Source: CAD feature listing. Evaluate the final solid. Frame: model axes, mm. Face numbers are marked on the shaded views. Round coordinates to 2 decimals unless told otherwise and drop trailing zeros. Order: outer loops, then holes, each group sorted by start corner. A loop starts at its lowest first (then second) coordinate and runs counter-clockwise, first axis right, second up. Notation, with made-up numbers: (65, 37.25) - (97, 37.25) arc R21 cw to (97, 45.25) - close; hole circle Ø1 at (-19, 30.5). An arc over 180 degrees is marked (long way). Put each result on its own line as item: value. Start each with the question number.
1) Line query: probe 1 along Y at (x, z) = (0, 14); probe 2 along X at (y, z) = (11, -13); probe 3 along X at (y, z) = (-3.25, 30). Output: solid intervals per line, ascending. Write a range as [from, to].
2) Contact query for flat-ended pins moving along their axis: P1, Ø8, axis at x = -0.5, z = 25.5, coming from the +Y side; P2, Ø6, axis at x = -10, y = 9, coming from the -Z side; P3, Ø1.5, axis at x = 9.5, z = 16, coming from the -Y side; P4, Ø4, axis at x = -9, z = 26, coming from the -Y side. Output: stop coordinate, or through.
3) Section A-A on x = 0. Output: boundary loops of the cut face in (y, z) (3 decimals).
4) Mould query, pull axis Y, two halves, no side actions, for the marked faces 1 and 2. Classes: +Y half, -Y half, draft (parallel to the pull), parting line (faces both ways), or undercut.
5) Section C-C on z = 19. Output: boundary loops of the cut face in (x, y), then the cut area to 3 significant figures.
Autodesk Inventor part; units mm, degrees
ref_plane "YZ Plane" through (0, 0, 0) normal (1, 0, 0) x (0, 1, 0)
ref_plane "XZ Plane" through (0, 0, 0) normal (0, 1, 0) x (-1, 0, 0)
ref_plane "XY Plane" through (0, 0, 0) normal (0, 0, 1) x (1, 0, 0)
sketch "Sketch1" plane through (0, 0, 0) normal (0, 0, 1) x (1, 0, 0)
  circle A0 centre (0, 0) radius 6.35
  circle A1 centre (0, 0) radius 12.7
  dimension "d0" = 12.7
  dimension "d1" = 25.4
extrude "Extrusion1" add sketch "Sketch1" along normal mid plane 69.85
chamfer "Chamfer1" distance 2.5 angle 45 1 edges at (-12.7, 0, -34.925) measured on face at (10.3988, -1.5197, -34.925)
chamfer "Chamfer2" distance 2.5 angle 45 1 edges at (-12.7, 0, 34.925) measured on face at (10.3988, -1.5197, 34.925)
properties part number "Piston pin"
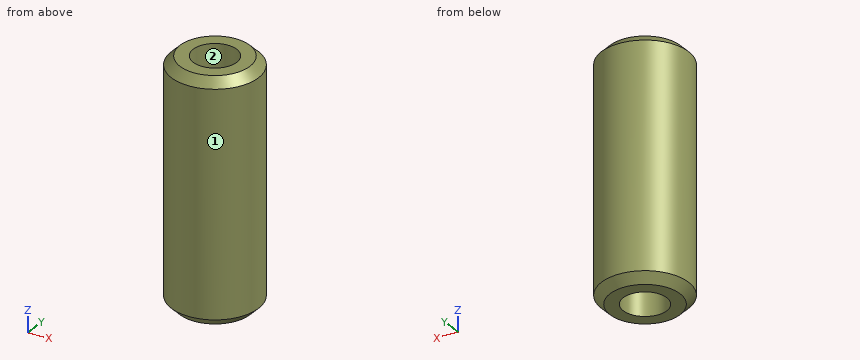
Answer sheet:
1. probe 1: [-12.7, -6.35], [6.35, 12.7]
1. probe 2: [-6.35, 6.35]
1. probe 3: [-12.28, -5.46], [5.46, 12.28]
2. P1: y = 12.7
2. P2: z = -34.67
2. P3: y = -9.2
2. P4: y = -10.6
3. outline: (-12.7, -32.425) - (-10.2, -34.925) - (-6.35, -34.925) - (-6.35, 34.925) - (-10.2, 34.925) - (-12.7, 32.425) - close; (6.35, -34.925) - (10.2, -34.925) - (12.7, -32.425) - (12.7, 32.425) - (10.2, 34.925) - (6.35, 34.925) - close
4. face 1: parting line
4. face 2: undercut
5. outline: circle Ø25.4 at (0, 0); hole circle Ø12.7 at (0, 0)
5. area: 380 mm^2
